```python
from build123d import *

# Parameters (mm, degrees)
ESQUISSE1_R                         = 3
BOSS_EXTRU_1_DEPTH                  = 27
DIAM_TRE_DU_PER_AGE_4_0_4_1_D       = 4
DIAM_TRE_DU_PER_AGE_4_0_4_1_DEPTH   = 24.5
DIAM_TRE_DU_PER_AGE_4_0_4_1_TIP     = 1.201721238
DIAM_TRE_DU_PER_AGE_2_5_2_5_2_D     = 2.5
DIAM_TRE_DU_PER_AGE_2_5_2_5_2_DEPTH = 3
DIAM_TRE_DU_PER_AGE_2_5_2_5_2_TIP   = 0.751075774
ENL_V_START                         = -15
ESQUISSE6_W                         = 11.750178357
ESQUISSE6_H                         = 11.384595502
ESQUISSE6_R                         = 2.5
ENL_V_MAT_EXTRU_1_DEPTH             = 6
CHANFREIN1_SIZE                     = 1
CHANFREIN2_SIZE                     = 0.75


with BuildPart() as part:
    # Esquisse1 → Boss.-Extru.1 (new body)
    with BuildSketch(Plane.XY):
        Circle(ESQUISSE1_R)
    extrude(amount=BOSS_EXTRU_1_DEPTH)

    # Diamètre du perçage Ø4.0 (4)1
    with Locations(Plane.XY.offset(27)):
        with Locations((0, 0)):
            Hole(DIAM_TRE_DU_PER_AGE_4_0_4_1_D / 2, depth=DIAM_TRE_DU_PER_AGE_4_0_4_1_DEPTH)
            with Locations((0, 0, -(DIAM_TRE_DU_PER_AGE_4_0_4_1_DEPTH + DIAM_TRE_DU_PER_AGE_4_0_4_1_TIP / 2))):  # 118° drill point
                Cone(0, DIAM_TRE_DU_PER_AGE_4_0_4_1_D / 2, DIAM_TRE_DU_PER_AGE_4_0_4_1_TIP, mode=Mode.SUBTRACT)

    # Diamètre du perçage Ø2.5 (2.5)2
    with Locations(Plane(origin=(0, 0, 0), x_dir=(-1, 0, 0), z_dir=(0, 0, -1))):
        with Locations((0, 0)):
            Hole(DIAM_TRE_DU_PER_AGE_2_5_2_5_2_D / 2, depth=DIAM_TRE_DU_PER_AGE_2_5_2_5_2_DEPTH)
            with Locations((0, 0, -(DIAM_TRE_DU_PER_AGE_2_5_2_5_2_DEPTH + DIAM_TRE_DU_PER_AGE_2_5_2_5_2_TIP / 2))):  # 118° drill point
                Cone(0, DIAM_TRE_DU_PER_AGE_2_5_2_5_2_D / 2, DIAM_TRE_DU_PER_AGE_2_5_2_5_2_TIP, mode=Mode.SUBTRACT)

    # Esquisse6 → Enlèv. mat.-Extru.1 (cut)
    with BuildSketch(Plane.XY.offset(27).offset(ENL_V_START)):
        with Locations((-0.219764127, 0.428836611)):
            Rectangle(ESQUISSE6_W, ESQUISSE6_H)
        Circle(ESQUISSE6_R, mode=Mode.SUBTRACT)
    extrude(amount=-ENL_V_MAT_EXTRU_1_DEPTH, mode=Mode.SUBTRACT)

    # Chanfrein1
    chanfrein1_edges = [part.edges().sort_by_distance(p)[0] for p in [
        (-3, 0, 0),
    ]]
    chamfer(chanfrein1_edges, length=CHANFREIN1_SIZE)

    # Chanfrein2
    # the kernel refuses this chamfer: 0.75 mm, written as the material it adds along each edge
    with BuildSketch(Plane(origin=(0, 0, 6), x_dir=(1, 0, 0), z_dir=(0, -1, 0))) as chanfrein2_piece_1_section:
        Polygon((2.5 + CHANFREIN2_SIZE, 0), (2.5, CHANFREIN2_SIZE), (2.5, 0), align=None)
    chanfrein2_piece_1 = revolve(axis=Axis((0, 0, 6), (0, 0, 1)), mode=Mode.PRIVATE)
    chanfrein2_piece_1 = chanfrein2_piece_1 & Plane(origin=(0, 0, 6.498848263), x_dir=(1, 0, 0), z_dir=(0, 0, -1)) * Cylinder(3, 13, mode=Mode.PRIVATE)
    add(chanfrein2_piece_1)


solid = part.part
```
Input: part model. Units: mm. Frame: model coordinates. A direction names the side the tool comes from. Coordinates: 2 decimals unless noted, no trailing zeros. Write each loop counter-clockwise with the first axis right and the second up, starting at its lowest first coordinate (ties: lowest second). Pieces come first, ordered by that corner, then holes. Notation, with made-up numbers: (-25, 27) - (18, 27) arc R12 ccw to (18, 43) - close; hole circle Ø4 at (-25.5, 82). An arc over 180 degrees is marked (long way). Put each result on its own line as item: value. Start each with the question number.
1) Reachability of faces 1 (the face through (-0.54, -2.44, 9.41)), 2 (the face through (0, -2, 15)), 3 (the face through (1, -2, 27)) from +Z, -Z, +X, -X, +Y, -Y: full face, straight path, thin tool, end or side. Return the list, or none.
2) Cut plane D-D (z = 20.5). Return the cut outline in (x, y), plus the area to 3 significant figures.
3) Contact query for flat-ended pins moving along their axis: pin 1 (3 mm diameter, centred on y = -1.5, z = 9, fed in from -X); pin 2 (2 mm diameter, centred on x = 0, y = 0, fed in from +Z); pin 3 (1 mm diameter, centred on y = 2.5, z = 4, fed in from -X). Output: stop coordinate, or through.
4) Ray query, L1, parallel to Y at x = 0, z = 19.25; L2, parallel to Y at x = 0, z = 0.5. Return the intervals inside material, ascending.
5) Mould query, pull axis X, two halves, no side actions, for faces 4 (the face through (-3, 0, 19)), 5 (the face through (-2, 2, 12)), 6 (the face through (0.672, 1.054, 1.039)). Classes: pulls with the +X half, pulls with the -X half, needs draft (parallel to the pull), parting line crosses it, or undercut.
6) Cut plane A-A (y = 0). Return the cut outline in (x, z), plus the area to 3 significant figures.
7) Cut plane C-C (z = 8.5). Return the cut outline in (x, y), plus the area to 3 significant figures.
Resolved:
1. face 1: none
1. face 2: +Z
1. face 3: +Z, +X, -X, +Y, -Y
2. outline: circle Ø6 at (0, 0); hole circle Ø4 at (0, 0)
2. area: 15.7 mm2
3. pin 1: stops at x = -2.5
3. pin 2: passes through
3. pin 3: stops at x = -2.24
4. L1: y = -3 to -2, 2 to 3
4. L2: y = -2.5 to -1.25, 1.25 to 2.5
5. face 4: parting line crosses it
5. face 5: needs draft
5. face 6: undercut
6. outline: (-3, 1) - (-2, 0) - (-1.25, 0) - (-1.25, 2.05) - (-2, 2.5) - (-2, 27) - (-3, 27) - (-3, 12) - (-2.5, 12) - (-2.5, 6.75) - (-3, 6.25) - close; (1.25, 0) - (2, 0) - (3, 1) - (3, 6.25) - (2.5, 6.75) - (2.5, 12) - (3, 12) - (3, 27) - (2, 27) - (2, 2.5) - (1.25, 2.05) - close
6. area: 50.9 mm2
7. outline: circle Ø5 at (0, 0); hole circle Ø4 at (0, 0)
7. area: 7.07 mm2
